from build123d import *

# Parameters (mm, degrees)
SKETCH1_W           = 70
SKETCH1_H           = 17
BOSS_EXTRUDE1_DEPTH = 3
SKETCH2_R           = 10.35
SKETCH2_R_2         = 1.559144978
BOSS_EXTRUDE2_DEPTH = 3
SKETCH3_R           = 1.6
CUT_EXTRUDE1_DEPTH  = 4
FILLET1_R           = 3
FILLET2_R           = 2


with BuildPart() as part:
    # Sketch1 → Boss-Extrude1 (new body)
    with BuildSketch(Plane(origin=(0, 0, 0), x_dir=(1, 0, 0), z_dir=(0, 1, 0))):
        with Locations((35, 8.5)):
            Rectangle(SKETCH1_W, SKETCH1_H)
    extrude(amount=BOSS_EXTRUDE1_DEPTH)

    # Sketch2 → Boss-Extrude2 (add)
    with BuildSketch(Plane.XY):
        with BuildLine():
            Line((0, 0), (70, 0))
            Line((70, 0), (70, 8))
            Line((70, 8), (51.37327089, 39.639294598))
            ThreePointArc((51.37327089, 39.639294598), (35, 49), (18.62672911, 39.639294598))
            Line((18.62672911, 39.639294598), (0, 8))
            Line((0, 8), (0, 0))
        make_face()
        with Locations((35, 30)):
            Circle(SKETCH2_R, mode=Mode.SUBTRACT)
        with Locations((35, 16)):
            Circle(SKETCH2_R_2, mode=Mode.SUBTRACT)
        with Locations((22.875644347, 37)):
            Circle(SKETCH2_R_2, mode=Mode.SUBTRACT)
        with Locations((47.124355653, 37)):
            Circle(SKETCH2_R_2, mode=Mode.SUBTRACT)
    extrude(amount=BOSS_EXTRUDE2_DEPTH)

    # Sketch3 → Cut-Extrude1 (cut, through all)
    with BuildSketch(Plane(origin=(0, 3, 0), x_dir=(1, 0, 0), z_dir=(0, 1, 0))):
        with Locations(Location((8.5, 8.5, 0), (0, 0, 270))):  # turned: the seam where the file's is
            Circle(SKETCH3_R)
        with Locations(Location((61.5, 8.5, 0), (0, 0, 270))):  # turned: the seam where the file's is
            Circle(SKETCH3_R)
    extrude(amount=-CUT_EXTRUDE1_DEPTH, mode=Mode.SUBTRACT)

    # Fillet1
    fillet1_edges = [part.edges().sort_by_distance(p)[0] for p in [
        (70, 1.5, -17),
        (0, 1.5, -17),
    ]]
    fillet(fillet1_edges, radius=FILLET1_R)

    # Fillet2
    fillet2_edges = [part.edges().sort_by_distance(p)[0] for p in [
        (35, 3, 0),
    ]]
    fillet(fillet2_edges, radius=FILLET2_R)


solid = part.part
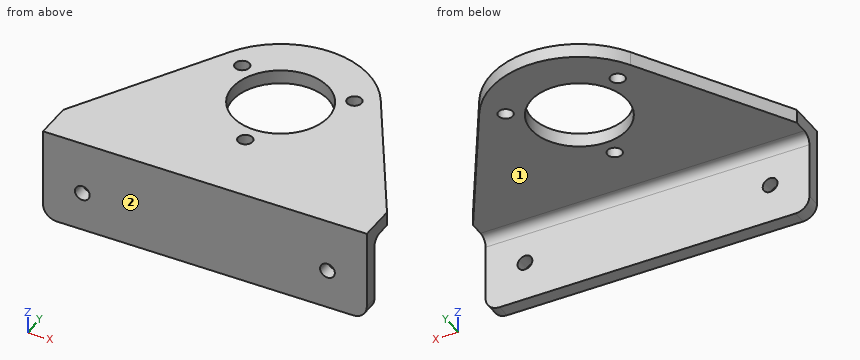
The model under review builds one solid part; all positions refer to its coordinate system, in mm. Face numbers are marked on the shaded views. A direction names the side the tool comes from. Give positions to 0.01 mm unless a question says otherwise; leave off trailing zeros. Write each loop counter-clockwise with the first axis right and the second up, starting at its lowest first coordinate (ties: lowest second). Pieces come first, ordered by that corner, then holes.
1. Add section B-B, the plane y = 30. Write out the cut boundary in (x, z), plus the area to 3 significant figures.
2. Add section D-D, the plane z = -11.5. Write out the cut boundary in (x, y), plus the area to 3 significant figures.
3. Wall thickness on L1, parallel to X at y = 2.1, z = -8.5; L2, parallel to Y at x = 17.5, z = -10.5: over which ranges is each line inside the solid? List them lowest first.
4. Add section C-C, the plane x = 61.5. Write out the cut boundary in (y, z), plus the area to 3 significant figures.
5. For P1, Ø2, axis at x = 22, y = 38.5, coming from the -Z side; P2, Ø3.5, axis at x = 61.5, z = -8.5, coming from the +Y side, all flat-tipped, find the tip position at first contact; note any pin that passes through.
6. Tool access review of the marked faces 1 and 2: name each direction out of +Z, -Z, +X, -X, +Y, -Y from which nothing blocks a thin tool from reaching the whole face with its end or side.
7. Add section A-A, the plane x = 35. Write out the cut boundary in (y, z), plus the area to 3 significant figures.
Worked answers:
1. outline: (12.95, 0) - (24.65, 0) - (24.65, 3) - (12.95, 3) - close; (45.35, 0) - (57.05, 0) - (57.05, 3) - (45.35, 3) - close
1. area: 70.2 mm2
2. outline: (0, 0) - (70, 0) - (70, 3) - (0, 3) - close
2. area: 210 mm2
3. L1: x = 0 to 6.9, 10.1 to 59.9, 63.1 to 70
3. L2: y = 0 to 3
4. outline: (0, -17) - (3, -17) - (3, -10.1) - (0, -10.1) - close; (0, -6.9) - (3, -6.9) - (3, -2) arc R2 cw to (5, 0) - (22.44, 0) - (22.44, 3) - (0, 3) - close
4. area: 110 mm2
5. P1: stops at z = 0
5. P2: stops at y = 3
6. face 1: -Z, +X, -X, +Y
6. face 2: +Z, -Z, +X, -X, -Y
7. outline: (0, -17) - (3, -17) - (3, -2) arc R2 cw to (5, 0) - (14.44, 0) - (14.44, 3) - (0, 3) - close; (17.56, 0) - (19.65, 0) - (19.65, 3) - (17.56, 3) - close; (40.35, 0) - (49, 0) - (49, 3) - (40.35, 3) - close
7. area: 127 mm2
